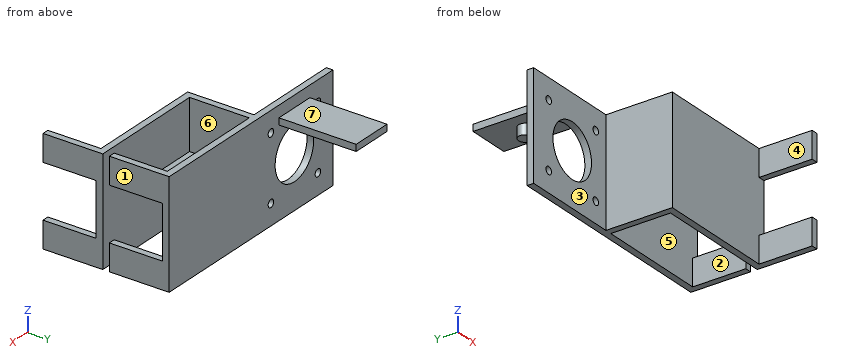
from build123d import *

# Parameters (mm, degrees)
SKETCH1_W            = 50.8
SKETCH1_H            = 50.8
BOSS_EXTRUDE1_DEPTH  = 3.175
SKETCH2_R            = 12.7
SKETCH2_R_2          = 1.8034
CUT_EXTRUDE1_DEPTH   = 37.061067996
SKETCH6_W            = 20.32
SKETCH6_H            = 3.175
BOSS_EXTRUDE4_DEPTH  = 36.9062
SKETCH7_R            = 3.1115
BOSS_EXTRUDE5_DEPTH  = 5.08
SKETCH11_W           = 3.175
SKETCH11_H           = 50.8
BOSS_EXTRUDE8_DEPTH  = 31.75
SKETCH13_W           = 50.8
SKETCH13_H           = 3.175
BOSS_EXTRUDE10_DEPTH = 57.15
SKETCH15_W           = 3.175
SKETCH15_H           = 12.7
BOSS_EXTRUDE12_DEPTH = 25.4
SKETCH16_W           = 3.175
SKETCH16_H           = 12.7
BOSS_EXTRUDE13_DEPTH = 25.4
SKETCH17_W           = 3.175
SKETCH17_H           = 28.575
BOSS_EXTRUDE14_DEPTH = 25.4


with BuildPart() as part:
    # Sketch1 → Boss-Extrude1 (new body)
    with BuildSketch(Plane(origin=(0, 0, 0), x_dir=(1, 0, 0), z_dir=(0, 1, 0))):
        Rectangle(SKETCH1_W, SKETCH1_H)
    extrude(amount=BOSS_EXTRUDE1_DEPTH)

    # Sketch2 → Cut-Extrude1 (cut, through all)
    with BuildSketch(Plane(origin=(0, 3.175, 0), x_dir=(1, 0, 0), z_dir=(0, 1, 0))):
        with Locations(Location((0, 0, 0), (0, 0, 270))):
            Circle(SKETCH2_R)
        with Locations(Location((-15.494, 15.494, 0), (0, 0, 270))):
            Circle(SKETCH2_R_2)
        with Locations(Location((15.494, 15.494, 0), (0, 0, 270))):
            Circle(SKETCH2_R_2)
        with Locations(Location((15.494, -15.494, 0), (0, 0, 270))):
            Circle(SKETCH2_R_2)
        with Locations(Location((-15.494, -15.494, 0), (0, 0, 270))):
            Circle(SKETCH2_R_2)
    extrude(amount=-CUT_EXTRUDE1_DEPTH, mode=Mode.SUBTRACT)

    # Sketch6 → Boss-Extrude4 (add)
    with BuildSketch(Plane(origin=(0, 3.175, 0), x_dir=(1, 0, 0), z_dir=(0, 1, 0))):
        with Locations((0, -18.2245)):
            Rectangle(SKETCH6_W, SKETCH6_H)
    extrude(amount=BOSS_EXTRUDE4_DEPTH)

    # Sketch7 → Boss-Extrude5 (add)
    with BuildSketch(Plane(origin=(0, 0, 16.637), x_dir=(-1, 0, 0), z_dir=(0, 0, -1))):
        with Locations(Location((1.27, 21.6281, 0), (0, 0, 180))):
            Circle(SKETCH7_R)
    extrude(amount=BOSS_EXTRUDE5_DEPTH)

    # Sketch11 → Boss-Extrude8 (add)
    with BuildSketch(Plane.XZ):
        with Locations((23.8125, 0)):
            Rectangle(SKETCH11_W, SKETCH11_H)
    extrude(amount=BOSS_EXTRUDE8_DEPTH)

    # Sketch13 → Boss-Extrude10 (add)
    with BuildSketch(Plane(origin=(25.4, 0, 0), x_dir=(0, 0, -1), z_dir=(1, 0, 0))):
        with Locations((0, -30.1625)):
            Rectangle(SKETCH13_W, SKETCH13_H)
        with Locations((0, 1.5875)):
            Rectangle(SKETCH13_W, SKETCH13_H)
    extrude(amount=BOSS_EXTRUDE10_DEPTH)

    # Sketch15 → Boss-Extrude12 (add)
    with BuildSketch(Plane.XZ.offset(31.75)):
        with Locations((80.9625, 19.05)):
            Rectangle(SKETCH15_W, SKETCH15_H)
        with Locations((80.9625, -19.05)):
            Rectangle(SKETCH15_W, SKETCH15_H)
    extrude(amount=BOSS_EXTRUDE12_DEPTH)

    # Sketch16 → Boss-Extrude13 (add)
    with BuildSketch(Plane.XZ):
        with Locations((80.9625, -19.05)):
            Rectangle(SKETCH16_W, SKETCH16_H)
        with Locations((80.9625, 19.05)):
            Rectangle(SKETCH16_W, SKETCH16_H)
    extrude(amount=BOSS_EXTRUDE13_DEPTH)

    # Sketch17 → Boss-Extrude14 (add)
    with BuildSketch(Plane(origin=(25.4, 0, 0), x_dir=(0, 0, -1), z_dir=(1, 0, 0))):
        with Locations((0, -14.2875)):
            Rectangle(SKETCH17_W, SKETCH17_H)
    extrude(amount=BOSS_EXTRUDE14_DEPTH)


solid = part.part
CAD build for the part. Positions are in the model's coordinates, mm. Face numbers are marked on the shaded views. A direction names the side the tool comes from. Give positions to 0.01 mm unless a question says otherwise; leave off trailing zeros. Loops run counter-clockwise (first coordinate to the right, second up) from the corner with the lowest first, then second, coordinate; pieces in that order, holes last. Notation, with made-up numbers: M 75.25,-33 L 82.25,-33 A26 ccw 82.25,-15 Z; hole C 74,-34.5 d9. An arc over 180 degrees is marked long. Answer in a Markdown table with one row per item. Add a question column.
Item 1: Band-saw the part on C-C on x = -1.27. Give the cut face in (y, z) (3 decimals), then the cut area to 3 significant figures.
Item 2: Band-saw the part on D-D on y = -19.5. Give the number of separate pieces and of enclosed holes in the cut face, then the cut area to 3 significant figures.
Item 3: Probe probe 1 along Y at (x, z) = (50, -15) (3 decimals); probe 2 along X at (y, z) = (-12.5, -20) (3 decimals); probe 3 along X at (y, z) = (1.15, 0). List the from-to ranges inside material, lowest first.
Item 4: Band-saw the part on A-A on y = -36. Give the cut face in (x, z) (3 decimals), then the cut area to 3 significant figures.
Item 5: Band-saw the part on B-B on z = 0. Give the cut face in (x, y) (3 decimals).
Item 6: Drop flat-ended pins along their axis: P1, Ø6.5, axis at y = -11.5, z = -20, coming from the -X side (3 decimals); P2, Ø10, axis at y = -40.5, z = 13.5, coming from the -X side (3 decimals); P3, Ø12, axis at y = 16.5, z = 14, coming from the -X side. Give the stop position or say it passes through.
Item 7: Tool access for the marked faces 4, 5, 6 and 7: list every direction of +Z, -Z, +X, -X, +Y, -Y with a clear straight run to the whole face (end or side of a thin tool).
Item 8: Mould opens along Y. For the marked faces 1, 2 and 3 say: +Y half, -Y half, draft (parallel to the pull), parting line (faces both ways), or undercut.
Reply:
| question | item | result |
|---|---|---|
| 1 | outline | M 0,-25.4 L 3.175,-25.4 L 3.175,-12.636 L 0,-12.636 Z; M 0,12.636 L 3.175,12.636 L 3.175,16.637 L 18.517,16.637 L 18.517,11.557 L 24.74,11.557 L 24.74,16.637 L 40.081,16.637 L 40.081,19.812 L 3.175,19.812 L 3.175,25.4 L 0,25.4 Z |
| 1 | area | 230 mm^2 |
| 2 | separate pieces | 3 |
| 2 | enclosed holes | 0 |
| 2 | area | 323 mm^2 |
| 3 | probe 1 | y = -31.75 to -28.575, 0 to 3.175 |
| 3 | probe 2 | x = 22.225 to 25.4, 79.375 to 82.55 |
| 3 | probe 3 | x = -25.4 to -12.7, 12.7 to 82.55 |
| 4 | outline | M 79.375,-25.4 L 82.55,-25.4 L 82.55,-12.7 L 79.375,-12.7 Z; M 79.375,12.7 L 82.55,12.7 L 82.55,25.4 L 79.375,25.4 Z |
| 4 | area | 80.6 mm^2 |
| 5 | outline | M -25.4,0 L -12.7,0 L -12.7,3.175 L -25.4,3.175 Z; M 12.7,0 L 22.225,0 L 22.225,-31.75 L 82.55,-31.75 L 82.55,-28.575 L 50.8,-28.575 L 50.8,0 L 82.55,0 L 82.55,3.175 L 12.7,3.175 Z |
| 6 | P1 | stops at x = 22.225 |
| 6 | P2 | stops at x = 79.375 |
| 6 | P3 | stops at x = -10.16 |
| 7 | face 4 | +Z, -Z, -X, -Y |
| 7 | face 5 | none |
| 7 | face 6 | +Z |
| 7 | face 7 | +Z, +X, -X, +Y |
| 8 | face 1 | draft |
| 8 | face 2 | undercut |
| 8 | face 3 | -Y half |
